```python
from build123d import *

# Parameters (mm, degrees)
F2_SIZE       = 0.81
F3_SIZE2      = 1.154701
F3_SIZE       = 2
F4_R          = 22.5
F5_DEPTH      = 50
F5_DEPTH_BACK = 16.8


with BuildPart() as f1:
    # F0 (on Front) → F1 (revolve)
    with BuildSketch(Plane.XZ):
        Polygon((0, 0), (0, -23.5), (65, -23.5), (65, -3.5), (60.5, -3.5), (60.5, 0), (49, 0), (49, -3.3), (33.6, -3.3), (33.6, 5), (0, 5), align=None)
    revolve(axis=Axis((0, 0, 20), (0, 0, 1)))

    # F2
    f2_edges = [f1.edges().sort_by_distance(p)[0] for p in [
        (-60.5, 0, 0),
    ]]
    chamfer(f2_edges, length=F2_SIZE)

    # F3
    f3_edges = [f1.edges().sort_by_distance(p)[0] for p in [
        (-33.6, 0, 5),
    ]]
    chamfer(f3_edges, length=F3_SIZE, length2=F3_SIZE2)


with BuildPart() as f5:
    # F4 (on face) → F5 (new body, two sides)
    with BuildSketch(Plane.XY.offset(5)) as f5_sk:
        Circle(F4_R)
    extrude(amount=-F5_DEPTH)
    extrude(f5_sk.sketch, amount=-F5_DEPTH_BACK)


with BuildPart() as f1_1:
    add(f1.part)

    # F6: cut F5
    add(f5.part, mode=Mode.SUBTRACT)


solid = f1_1.part
```
Design review of the part built by this model. Coordinates are the model's own, in mm. A direction names the side the tool comes from. Coordinates: 2 decimals unless noted, no trailing zeros. Order: outer loops, then holes, each group sorted by start corner. A loop starts at its lowest first (then second) coordinate and runs counter-clockwise, first axis right, second up. Notation, with made-up numbers: (25.5, -35) - (82.5, -35) arc R25 ccw to (82.5, -5) - close; hole circle Ø11 at (-4.5, 16.5). An arc over 180 degrees is marked (long way). Answer in a Markdown table with one row per item.
(1) Consider section C-C on z = -12. State the section outline as (x, y) points, plus the area to 3 significant figures.
Checked values:
| item | result |
|---|---|
| outline | circle Ø130 at (0, 0); hole circle Ø45 at (0, 0) |
| area | 11,700 mm^2 |
(2) Consider section A-A on y = 0. State the section outline as (x, z) points, plus the area to 3 significant figures.
Checked values:
| item | result |
|---|---|
| outline | (-65, -23.5) - (-22.5, -23.5) - (-22.5, 5) - (-32.45, 5) - (-33.6, 3) - (-33.6, -3.3) - (-49, -3.3) - (-49, 0) - (-59.69, 0) - (-60.5, -0.81) - (-60.5, -3.5) - (-65, -3.5) - close; (22.5, -23.5) - (65, -23.5) - (65, -3.5) - (60.5, -3.5) - (60.5, -0.81) - (59.69, 0) - (49, 0) - (49, -3.3) - (33.6, -3.3) - (33.6, 3) - (32.45, 5) - (22.5, 5) - close |
| area | 1,970 mm^2 |
(3) Wall thickness on line 1 along Y through (x, z) = (0, -1.15); line 2 along Y through (x, z) = (0, -7.75); line 3 along Z through (x, y) = (-9.5, 57.5): over which ranges is each line inside the solid? List them lowest first. Write a range as from..to.
Checked values:
| item | result |
|---|---|
| line 1 | -60.5..-49, -33.6..-22.5, 22.5..33.6, 49..60.5 |
| line 2 | -65..-22.5, 22.5..65 |
| line 3 | -23.5..0 |
(4) Clearance check with flat-ended pins moving along their axes: pin 1 (2 mm diameter, centred on y = -48.5, z = -7.5, fed in from -X); pin 2 (10 mm diameter, centred on x = -39.5, z = -3, fed in from +Y); pin 3 (1.5 mm diameter, centred on x = -13.5, z = -12.5, fed in from +Y). State where each tip first meets the part, or that it passes through.
Checked values:
| item | result |
|---|---|
| pin 1 | x = -44.37 |
| pin 2 | y = 55.07 |
| pin 3 | y = 63.74 |
(5) The part is to be moulded in two halves that separate along X. For faces 1 (the cylindrical face through (10.382, -19.961, -9.05)), 2 (the cylindrical face through (-13.12, -59.06, -2.14)), 3 (the flat face through (-22, -7, 5)), say which applies: released by +X, released by -X, zero draft, split by the parting line, or undercut.
Checked values:
| item | result |
|---|---|
| face 1 | undercut |
| face 2 | split by the parting line |
| face 3 | zero draft |
(6) For faces 4 (the cylindrical face through (32.05, 10.09, -0.11)), 5 (the flat face through (-28, 1, -23.5)), list the 3-axis set-ups (+Z, -Z, +X, -X, +Y, -Y) from which the entire face can be reached by the end or side of a thin tool; tool diameter is ignored.
Checked values:
| item | result |
|---|---|
| face 4 | +Z |
| face 5 | -Z, +X, -X, +Y, -Y |
